The listing builds one solid part. Answer for the finished solid, in the listing's coordinates (mm). A direction names the side the tool comes from. Coordinates: 2 decimals unless noted, no trailing zeros. Write each loop counter-clockwise with the first axis right and the second up, starting at its lowest first coordinate (ties: lowest second). Pieces come first, ordered by that corner, then holes.
Autodesk Inventor part; units mm, degrees
ref_plane "YZ Plane" through (0, 0, 0) normal (1, 0, 0) x (0, 1, 0)
ref_plane "XZ Plane" through (0, 0, 0) normal (0, 1, 0) x (-1, 0, 0)
ref_plane "XY Plane" through (0, 0, 0) normal (0, 0, 1) x (1, 0, 0)
sketch "Sketch5" plane through (0, 0, 0) normal (0, 1, 0) x (-1, 0, 0)
  line L0 (0, 0) -> (180, 0)
  line L1 (180, 0) -> (180, -12)
  line L2 (0, -12) -> (0, 0)
  line L3 (166, -26) -> (14, -26)
  line L4 (0, -12) -> (14, -26)
  line L5 (180, -12) -> (166, -26)
  circle A0 centre (101, -18) radius 3
  circle A1 centre (79, -18) radius 3
  circle A2 centre (57, -18) radius 3
  circle A3 centre (123, -18) radius 3
  circle A4 centre (145, -18) radius 3
  circle A5 centre (35, -18) radius 3
  dimension "d57" = 6
  dimension "d58" = 79
  dimension "d59" = 180
  dimension "d60" = 12
  dimension "d61" = 14
  dimension "d62" = 14
  dimension "d63" = 14
  dimension "d64" = 14
  dimension "d65" = 152
  dimension "d66" = 8
  dimension "d67" = 6
  dimension "d68" = 6
  dimension "d69" = 6
  dimension "d70" = 6
  dimension "d71" = 8
  dimension "d72" = 8
  dimension "d73" = 8
  dimension "d74" = 8
  dimension "d75" = 22
  dimension "d76" = 22
  dimension "d77" = 22
  dimension "d78" = 22
  dimension "d95" = 6
  dimension "d96" = 0
  dimension "d97" = 22
extrude "Extrusion7" add sketch "Sketch5" along normal blind 12
sketch "Sketch8" plane through (0, 0, 0) normal (0, -1, 0) x (1, 0, 0)
  line L0 (0, 0) -> (0, -12)
  line L1 (0, 0) -> (-12, 0)
  line L2 (-12, 0) -> (-12, -12)
  line L3 (-12, -12) -> (0, -12)
  line L4 (0, -12) -> (0, 0)
  line L5 (-180, -12) -> (-180, 0)
  line L6 (-180, 0) -> (-168, 0)
  line L7 (-168, 0) -> (-168, -12)
  line L8 (-168, -12) -> (-180, -12)
  line L9 (-180, -12) -> (-180, 0)
  dimension "d100" = 12
  dimension "d101" = 12
  dimension "d102" = 12
  dimension "d103" = 12
extrude "Extrusion8" add sketch "Sketch8" along normal blind 12
sketch "Sketch11" plane through (0, 12, 0) normal (0, 1, 0) x (1, 0, 0)
  circle A0 centre (-35, 18) radius 3
  line L0 (-38.0022, 12.8) -> (-41.0044, 18)
  line L1 (-41.0044, 18) -> (-38.0022, 23.2)
  line L2 (-38.0022, 23.2) -> (-31.9978, 23.2)
  line L3 (-31.9978, 23.2) -> (-28.9956, 18)
  line L4 (-28.9956, 18) -> (-31.9978, 12.8)
  line L5 (-31.9978, 12.8) -> (-38.0022, 12.8)
  circle A1 centre (-57, 18) radius 3
  line L6 (-60.0022, 12.8) -> (-63.0044, 18)
  line L7 (-63.0044, 18) -> (-60.0022, 23.2)
  line L8 (-60.0022, 23.2) -> (-53.9978, 23.2)
  line L9 (-53.9978, 23.2) -> (-50.9956, 18)
  line L10 (-50.9956, 18) -> (-53.9978, 12.8)
  line L11 (-53.9978, 12.8) -> (-60.0022, 12.8)
  line L12 (-75.9978, 12.8) -> (-82.0022, 12.8)
  line L13 (-82.0022, 12.8) -> (-85.0044, 18)
  line L14 (-85.0044, 18) -> (-82.0022, 23.2)
  line L15 (-82.0022, 23.2) -> (-75.9978, 23.2)
  line L16 (-75.9978, 23.2) -> (-72.9956, 18)
  line L17 (-72.9956, 18) -> (-75.9978, 12.8)
  circle A2 centre (-101, 18) radius 3
  line L18 (-104.0022, 12.8) -> (-107.0044, 18)
  line L19 (-107.0044, 18) -> (-104.0022, 23.2)
  line L20 (-104.0022, 23.2) -> (-97.9978, 23.2)
  line L21 (-97.9978, 23.2) -> (-94.9956, 18)
  line L22 (-94.9956, 18) -> (-97.9978, 12.8)
  line L23 (-97.9978, 12.8) -> (-104.0022, 12.8)
  circle A3 centre (-123, 18) radius 3
  line L24 (-119.9978, 12.8) -> (-126.0022, 12.8)
  line L25 (-126.0022, 12.8) -> (-129.0044, 18)
  line L26 (-129.0044, 18) -> (-126.0022, 23.2)
  line L27 (-126.0022, 23.2) -> (-119.9978, 23.2)
  line L28 (-119.9978, 23.2) -> (-116.9956, 18)
  line L29 (-116.9956, 18) -> (-119.9978, 12.8)
  circle A4 centre (-145, 18) radius 3
  line L30 (-148.0022, 12.8) -> (-151.0044, 18)
  line L31 (-151.0044, 18) -> (-148.0022, 23.2)
  line L32 (-148.0022, 23.2) -> (-141.9978, 23.2)
  line L33 (-141.9978, 23.2) -> (-138.9956, 18)
  line L34 (-138.9956, 18) -> (-141.9978, 12.8)
  line L35 (-141.9978, 12.8) -> (-148.0022, 12.8)
  point P0 (0, 0)
  point P1 (-79, 18)
  dimension "d123" = 5.2
  dimension "d125" = 5.2
  dimension "d126" = 5.2
  dimension "d127" = 5.2
  dimension "d128" = 5.2
  dimension "d129" = 22
extrude "Extrusion11" cut sketch "Sketch11" against normal blind 5
hole "Hole3" at (-6, -6, 0) direction (0, 0, -1) diameter 6.4 depth 12 tip angle 118
hole "Hole4" at (-174, -6, 0) direction (0, 0, -1) diameter 6.4 depth 12 tip angle 118
properties part number "frameBottomRight" material "ABS Plastic"
1. Section B-B on z = -6 is taken. Give the vertices of the cut face in (x, y).
Results found:
outline: (-180, -12) - (-168, -12) - (-168, 0) - (-12, 0) - (-12, -12) - (0, -12) - (0, 12) - (-180, 12) - close; hole circle Ø6.4 at (-174, -6); hole circle Ø6.4 at (-6, -6)
2. Section D-D on x = -6 is taken. Give the vertices of the cut face in (y, z), then the cut area to 3 significant figures.
Results found:
outline: (-12, -12) - (-9.2, -12) - (-9.2, 0) - (-12, 0) - close; (-2.8, -12) - (0, -12) - (0, -18) - (12, -18) - (12, 0) - (-2.8, 0) - close
area: 283 mm2
3. Find the intervals of material crossed by L1, parallel to X at y = -6, z = -4.75; L2, parallel to X at y = -9.5, z = -1.75; L3, parallel to Y at x = -17.5, z = -17, in increasing order.
Results found:
L1: x = -180 to -177.2, -170.8 to -168, -12 to -9.2, -2.8 to 0
L2: x = -180 to -168, -12 to 0
L3: y = 0 to 12
4. A tool of negligible diameter and unlimited length cuts with its end or side. For faces 1 (the cylindrical face through (-98.6, 3.5, -16.2)), 2 (the cylindrical face through (-2.876, -5.306, -6.084)), 3 (the flat face through (-12, -6, -6)), 4 (the flat face through (-171, -3, -12)), 5 (the flat face through (-61.524, 9.535, -20.564)), from which of +Z, -Z, +X, -X, +Y, -Y can it reach the whole face along a straight path? Write none if from no direction.
Results found:
face 1: +Y, -Y
face 2: +Z, -Z
face 3: +Z, -Z, -Y
face 4: -Z, +X, -X, -Y
face 5: +Y
5. Section C-C on y = -7.25 is taken. Give the vertices of the cut face in (x, z), then the cut area to 3 significant figures.
Results found:
outline: (-180, -12) - (-176.95, -12) - (-176.95, 0) - (-180, 0) - close; (-171.05, -12) - (-168, -12) - (-168, 0) - (-171.05, 0) - close; (-12, -12) - (-8.95, -12) - (-8.95, 0) - (-12, 0) - close; (-3.05, -12) - (0, -12) - (0, 0) - (-3.05, 0) - close
area: 147 mm2
6. For a pull along X with two mould halves and no side action, classify faces 6 (the flat face through (-89, 0, -13)), 7 (the flat face through (-89, 5, 0)) as pulls with the +X half, pulls with the -X half, needs draft (parallel to the pull), parting line crosses it, or undercut.
Results found:
face 6: undercut
face 7: needs draft
7. Section A-A on x = -57 is taken. Give the vertices of the cut face in (y, z), then the cut area to 3 significant figures.
Results found:
outline: (0, -26) - (12, -26) - (12, -23.2) - (7, -23.2) - (7, -21) - (0, -21) - close; (0, -15) - (7, -15) - (7, -12.8) - (12, -12.8) - (12, 0) - (0, 0) - close
area: 218 mm2
8. Flat-ended cylindrical pins translate along their axes: P1, Ø1, axis at y = 7.5, z = -11.5, coming from the +X side; P2, Ø8, axis at y = 1, z = -21, coming from the -X side. Find the tip coordinate at first contact, or state that the pin passes through.
Results found:
P1: stops at x = 0
P2: stops at x = -175
